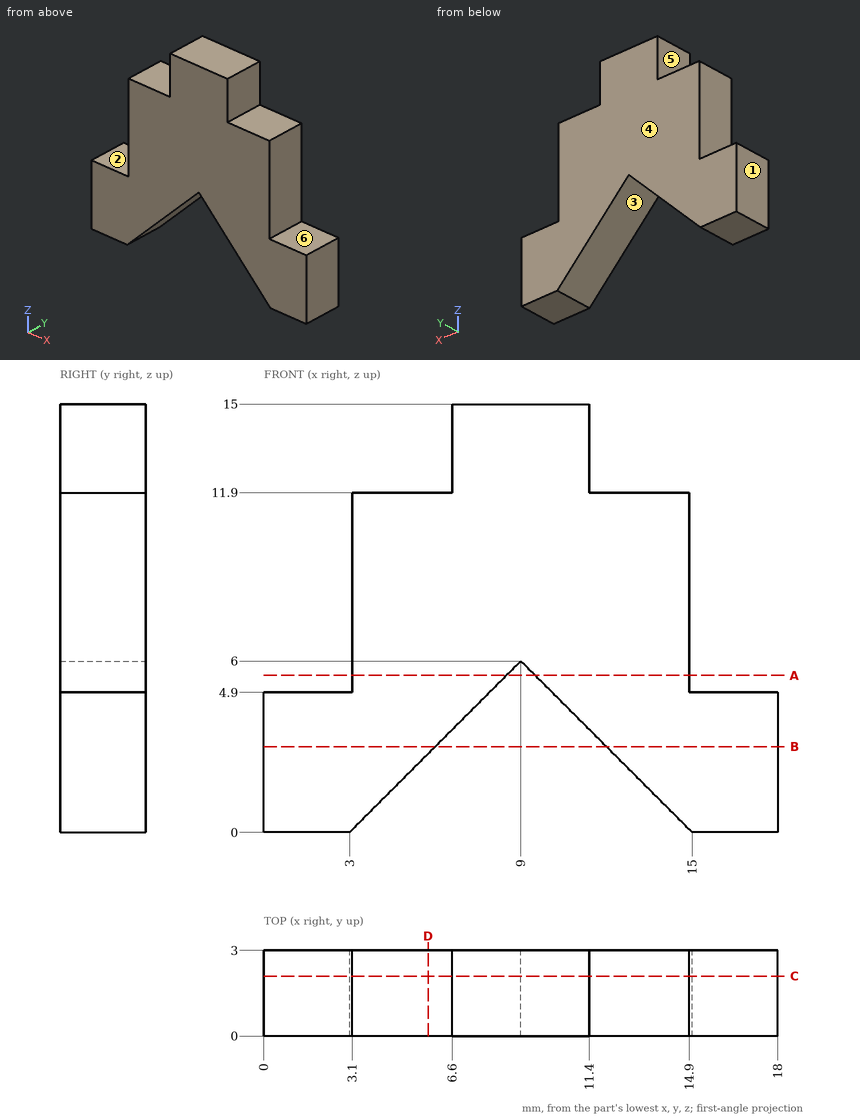
Part print with two shaded views. Sizes in mm from the minimum x, y, z corner. A direction names the side the tool comes from. Round coordinates to 2 decimals unless told otherwise and drop trailing zeros. Order: outer loops, then holes, each group sorted by start corner. A loop starts at its lowest first (then second) coordinate and runs counter-clockwise, first axis right, second up. Notation, with made-up numbers: (66.25, 72.25) - (122.25, 72.25) arc R28 ccw to (122.25, 94.25) - close; hole circle Ø8 at (53.25, 6). An arc over 180 degrees is marked (long way). Return JSON: item names as keys, results as strings.
(1) Cut at B-B (z = 3). Give the cut face in (x, y).
Answer key:
{"outline": "(0, 0) - (6, 0) - (6, 3) - (0, 3) - close; (12, 0) - (18, 0) - (18, 3) - (12, 3) - close"}
(2) Wall check: probe 1 along X at (y, z) = (2.85, 9); probe 2 along X at (y, z) = (2.85, 4); probe 3 along Z at (x, y) = (16.5, 1.6). Give the ranges that are in metal, low to high. Write a range as from..to.
Answer key:
{"probe 1": "x = 3.1..14.9", "probe 2": "x = 0..7, 11..18", "probe 3": "z = 0..4.9"}
(3) Pull direction X, two halves, no side cores. Call the marked faces 1, 2 and 3: +X half, -X half, draft (parallel to the pull), parting line (faces both ways), or undercut.
Answer key:
{"face 1": "-X half", "face 2": "draft", "face 3": "undercut"}
(4) Cut at A-A (z = 5.5). Give the cut face in (x, y).
Answer key:
{"outline": "(3.1, 0) - (8.5, 0) - (8.5, 3) - (3.1, 3) - close; (9.5, 0) - (14.9, 0) - (14.9, 3) - (9.5, 3) - close"}
(5) Pin check, flat tips, straight feed: pin 1 Ø1 at (y, z) = (2.5, 13.5) entering from -X; pin 2 Ø0.9 at (x, y) = (16.5, 2) entering from +Z; pin 3 Ø1 at (y, z) = (2, 11) entering from +X. Stop position of each tip, or through.
Answer key:
{"pin 1": "stops at x = 6.6", "pin 2": "stops at z = 4.9", "pin 3": "stops at x = 14.9"}
(6) Cut at C-C (y = 2.1). Give the cut face in (x, z), then the cut area to 3 significant figures.
Answer key:
{"outline": "(0, 0) - (3, 0) - (9, 6) - (15, 0) - (18, 0) - (18, 4.9) - (14.9, 4.9) - (14.9, 11.9) - (11.4, 11.9) - (11.4, 15) - (6.6, 15) - (6.6, 11.9) - (3.1, 11.9) - (3.1, 4.9) - (0, 4.9) - close", "area": "150 mm^2"}
(7) Cut at D-D (x = 5.75). Give the cut face in (y, z).
Answer key:
{"outline": "(0, 2.75) - (3, 2.75) - (3, 11.9) - (0, 11.9) - close"}
(8) Tool access for the marked faces 4, 5 and 6: list every direction of +Z, -Z, +X, -X, +Y, -Y with a clear straight run to the whole face (end or side of a thin tool).
Answer key:
{"face 4": "+Z, -Z, +X, -X, +Y", "face 5": "+Z, -X, +Y, -Y", "face 6": "+Z, +X, +Y, -Y"}
